CAD build for the part. Positions are in the model's coordinates, mm. Face numbers are marked on the shaded views. A direction names the side the tool comes from. Round coordinates to 2 decimals unless told otherwise and drop trailing zeros. Loops run counter-clockwise (first coordinate to the right, second up) from the corner with the lowest first, then second, coordinate; pieces in that order, holes last.
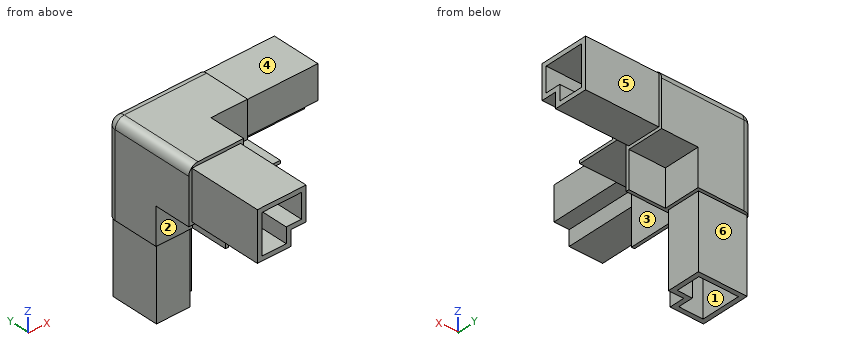
```python
from build123d import *

# Parameters (mm, degrees)
F1_DEPTH  = 50
F3_DEPTH  = 50
F5_DEPTH  = 50
F7_DEPTH  = 90
F9_DEPTH  = 90
F11_DEPTH = 90
F12_R     = 5


with BuildPart() as f1:
    # F0 (on Front) → F1 (new body)
    with BuildSketch(Plane.XZ):
        Polygon((30, 0), (0, 0), (0, -30), (20, -30), (20, -50), (21.7, -50), (21.7, -21.7), (50, -21.7), (50, -20), (30, -20), align=None)
        Polygon((28.3, -20), (20, -20), (20, -28.3), (1.7, -28.3), (1.7, -1.7), (28.3, -1.7), align=None, mode=Mode.SUBTRACT)
    extrude(amount=F1_DEPTH)

    # F2 (on Right) → F3 (join)
    with BuildSketch(Plane.YZ):
        Polygon((0, -30), (0, 0), (-30, 0), (-30, -20), (-50, -20), (-50, -21.7), (-21.7, -21.7), (-21.7, -50), (-20, -50), (-20, -30), align=None)
        Polygon((-28.3, -1.7), (-1.7, -1.7), (-1.7, -28.3), (-20, -28.3), (-20, -20), (-28.3, -20), align=None, mode=Mode.SUBTRACT)
    extrude(amount=F3_DEPTH)

    # F4 (on face) → F5 (join)
    with BuildSketch(Plane.XY):
        Polygon((30, 0), (0, 0), (0, -30), (20, -30), (20, -50), (21.7, -50), (21.7, -21.7), (50, -21.7), (50, -20), (30, -20), align=None)
        Polygon((28.3, -20), (20, -20), (20, -28.3), (1.7, -28.3), (1.7, -1.7), (28.3, -1.7), align=None, mode=Mode.SUBTRACT)
    extrude(amount=-F5_DEPTH)

    # F6 (on face) → F7 (join)
    with BuildSketch(Plane(origin=(0, 0, 0), x_dir=(0, -1, 0), z_dir=(-1, 0, 0))):
        Polygon((20, -1.7), (1.7, -1.7), (1.7, -20), (1.7, -21.7), (1.7, -28.3), (20, -28.3), (20, -21.7), (20, -20), (21.7, -20), (28.3, -20), (28.3, -1.7), (21.7, -1.7), align=None)
        Polygon((4.2, -20), (4.2, -4.2), (20, -4.2), (21.7, -4.2), (25.8, -4.2), (25.8, -17.5), (21.7, -17.5), (17.5, -17.5), (17.5, -21.7), (17.5, -25.8), (4.2, -25.8), (4.2, -21.7), align=None, mode=Mode.SUBTRACT)
    extrude(amount=-F7_DEPTH)

    # F8 (on face) → F9 (join)
    with BuildSketch(Plane(origin=(0, 0, 0), x_dir=(-1, 0, 0), z_dir=(0, 1, 0))):
        Polygon((-1.7, -20), (-1.7, -1.7), (-20, -1.7), (-21.7, -1.7), (-28.3, -1.7), (-28.3, -20), (-21.7, -20), (-20, -20), (-20, -21.7), (-20, -28.3), (-1.7, -28.3), (-1.7, -21.7), align=None)
        Polygon((-20, -4.2), (-4.2, -4.2), (-4.2, -20), (-4.2, -21.7), (-4.2, -25.8), (-17.5, -25.8), (-17.5, -21.7), (-17.5, -17.5), (-21.7, -17.5), (-25.8, -17.5), (-25.8, -4.2), (-21.7, -4.2), align=None, mode=Mode.SUBTRACT)
    extrude(amount=-F9_DEPTH)

    # F10 (on face) → F11 (join)
    with BuildSketch(Plane.XY):
        Polygon((20, -1.7), (1.7, -1.7), (1.7, -20), (1.7, -21.7), (1.7, -28.3), (20, -28.3), (20, -21.7), (20, -20), (21.7, -20), (28.3, -20), (28.3, -1.7), (21.7, -1.7), align=None)
        Polygon((4.2, -25.8), (4.2, -21.7), (4.2, -20), (4.2, -4.2), (20, -4.2), (21.7, -4.2), (25.8, -4.2), (25.8, -17.5), (21.7, -17.5), (17.5, -17.5), (17.5, -21.7), (17.5, -25.8), align=None, mode=Mode.SUBTRACT)
    extrude(amount=-F11_DEPTH)

    # F12
    f12_edges = [f1.edges().sort_by_distance(p)[0] for p in [
        (0, -25, 0),
        (0, 0, -25),
        (25, 0, 0),
    ]]
    fillet(f12_edges, radius=F12_R)


solid = f1.part
```
Item 1: Two-plate mould, pull along X, no slides. Class the marked faces 1, 2 and 3: released by +X, released by -X, zero draft, split by the parting line, or undercut.
Answers follow:
face 1: undercut
face 2: zero draft
face 3: released by +X
Item 2: Cut at B-B, the plane y = -46.5. Give the cut face in (x, z), plus the area to 3 significant figures.
Answers follow:
outline: (0, -30) - (20, -30) - (20, -50) - (21.7, -50) - (21.7, -21.7) - (50, -21.7) - (50, -20) - (30, -20) - (30, 0) - (5, 0) arc R5 ccw to (0, -5) - close; hole (4.2, -25.8) - (17.5, -25.8) - (17.5, -21.7) - (4.2, -21.7) - close; hole (4.2, -20) - (17.5, -20) - (17.5, -17.5) - (20, -17.5) - (20, -4.2) - (4.2, -4.2) - close; hole (21.7, -17.5) - (25.8, -17.5) - (25.8, -4.2) - (21.7, -4.2) - close
area: 541 mm2
Item 3: Probe line 1 (Y direction, x = 12, z = -25); line 2 (Y direction, x = 17, z = -38.5). List the from-to ranges inside material, lowest first.
Answers follow:
line 1: y = -30 to -25.8, -21.7 to -17.5, -4.2 to 0
line 2: y = -30 to -25.8, -21.7 to -20, -4.2 to 0
Item 4: 3-axis set-ups, long thin cutter, end or side, ignore diameter. For the marked faces 4, 5 and 6: which of +Z, -Z, +X, -X, +Y, -Y reach the whole face in a straight line?
Answers follow:
face 4: +Z, +X, +Y, -Y
face 5: +Z, -Z, +X, +Y
face 6: -Z, +X, -X, +Y
Item 5: Flat gauge pins, fed straight in: P1, Ø12, axis at x = 72.5, y = -30.5, coming from the +Z side; P2, Ø10.5, axis at x = 37, z = -7.5, coming from the -Y side; P3, Ø9, axis at x = 64.5, y = -8, coming from the -Z side. Where does each tip first touch, or does it go through?
Answers follow:
P1: stops at z = -1.7
P2: stops at y = -30
P3: stops at z = -28.3
Item 6: Cut at D-D, the plane x = 59.5. Give the cut face in (y, z), plus the area to 3 significant figures.
Answers follow:
outline: (-28.3, -20) - (-20, -20) - (-20, -28.3) - (-1.7, -28.3) - (-1.7, -1.7) - (-28.3, -1.7) - close; hole (-25.8, -17.5) - (-17.5, -17.5) - (-17.5, -25.8) - (-4.2, -25.8) - (-4.2, -4.2) - (-25.8, -4.2) - close
area: 241 mm2
Item 7: Cut at A-A, the plane z = -79. Give the cut face in (x, y), plus the area to 3 significant figures.
Answers follow:
outline: (1.7, -28.3) - (20, -28.3) - (20, -20) - (28.3, -20) - (28.3, -1.7) - (1.7, -1.7) - close; hole (4.2, -25.8) - (17.5, -25.8) - (17.5, -17.5) - (25.8, -17.5) - (25.8, -4.2) - (4.2, -4.2) - close
area: 241 mm2
